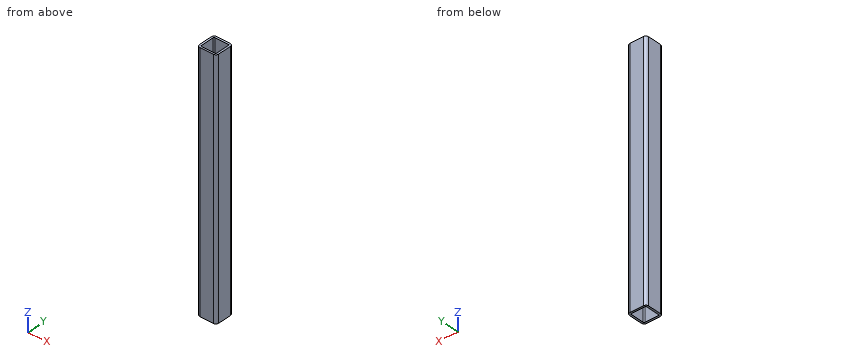
Autodesk Inventor part; units mm, degrees
ref_plane "Start Plane" through (0, 0, 10) normal (0, 0, 1) x (1, 0, 0)
ref_plane "End Plane" through (0, 0, 270) normal (0, 0, 1) x (1, 0, 0)
ref_plane "Work Plane4" through (167.5, -7, 270) normal (0, 0, 1) x (1, 0, 0)
ref_plane "Start Plane" through (0, 0, 10) normal (0, 0, 1) x (1, 0, 0)
ref_plane "End Plane" through (0, 0, 270) normal (0, 0, 1) x (1, 0, 0)
sketch "Sketch" plane through (0, 0, 0) normal (0, 0, 1) x (1, 0, 0)
  line L0 (-10, -7) -> (-10, 7)
  line L1 (-7, 10) -> (7, 10)
  line L2 (10, 7) -> (10, -7)
  line L3 (7, -10) -> (-7, -10)
  arc A0 (-10, -7) -> (-7, -10) centre (-7, -7) ccw
  arc A1 (-7, 10) -> (-10, 7) centre (-7, 7) ccw
  arc A2 (10, 7) -> (7, 10) centre (7, 7) ccw
  arc A3 (7, -10) -> (10, -7) centre (7, -7) ccw
  arc A4 (-7, 8) -> (-8, 7) centre (-7, 7) ccw
  line L4 (-7, 8) -> (7, 8)
  arc A5 (8, 7) -> (7, 8) centre (7, 7) ccw
  line L5 (8, 7) -> (8, -7)
  arc A6 (7, -8) -> (8, -7) centre (7, -7) ccw
  line L6 (7, -8) -> (-7, -8)
  arc A7 (-8, -7) -> (-7, -8) centre (-7, -7) ccw
  line L7 (-8, -7) -> (-8, 7)
  line L8 (0, 14.8698) -> (0, -14.8698) construction
  line L9 (-14.8698, 0) -> (14.8698, 0) construction
  dimension "d7" = 3
  dimension "d10" = 20
  dimension "d11" = 20
  dimension "d12" = 2
  dimension "d15" = 10
  dimension "d16" = 10
extrude "Body" add sketch "Sketch" along normal up to surface (260 mm away) from surface at 10
sketch "Sketch3" plane through (0, 0, 0) normal (0, 0, 1) x (1, 0, 0)
  line L0 (0, 0) -> (10, 0)
ref_plane "Work Plane3" through (0, 0, 0) normal (0, -1, 0) x (1, 0, 0)
sketch "Sketch4" plane through (0, 0, 0) normal (0, -1, 0) x (1, 0, 0)
  line L0 (-2, 10) -> (12, 10)
  line L1 (-2, 270) -> (12, 270)
  dimension "d18" = 260
ref_plane "Work Plane4" through (167.5, -7, 270) normal (0, 0, 1) x (1, 0, 0)
split "Split1" plane through (167.5, -7, 270) removes the side toward (0, 0, 1)
ref_plane "Work Plane5" through (-75, -7, 10) normal (0, 0, -1) x (-1, 0, 0)
split "Split2" plane through (-75, -7, 10) removes the side toward (0, 0, -1)
equation "\"d7\" = G_IR"
equation "\"d10\" = G_H"
equation "\"d11\" = G_W"
equation "\"d12\" = G_T"
equation "\"d15\" = 0.5 * d10"
equation "\"d16\" = 0.5 * d11"
equation "\"d3\" = G_L"
equation "\"G_W\" = 20"
equation "\"G_H\" = 20"
equation "\"G_T\" = 2"
equation "\"G_IR\" = 3"
equation "\"G_L\" = d18"
properties part number "ISO 12633-2 - 20x20x2 - 260" material "Steel, Mild"
The model under review builds one solid part; all positions refer to its coordinate system, in mm. Give positions to 0.01 mm unless a question says otherwise; leave off trailing zeros. Order: outer loops, then holes, each group sorted by start corner. A loop starts at its lowest first (then second) coordinate and runs counter-clockwise, first axis right, second up. Notation, with made-up numbers: (0, 24.25) - (11, 24.25) arc R12 cw to (11, 45.25) - close; hole circle Ø11 at (42.5, 42.5). An arc over 180 degrees is marked (long way). Use CSV: the item, a comma, the result in double quotes. Start each with the question number.
Q1. We need section A-A, the plane x = -3.75. Write out the cut boundary in (y, z), and give its area (3 significant figures).
Q2. We need section C-C, the plane z = 218. Write out the cut boundary in (x, y).
Q3. To check wall thickness, follow line 1 along Y through (x, z) = (4.5, 92.5); line 2 along X through (y, z) = (-7.5, 240.5). State the ranges of each line that lie inside material, in increasing order. Write a range as [from, to].
Outcome:
1,outline,"(-10, 10) - (-8, 10) - (-8, 270) - (-10, 270) - close; (8, 10) - (10, 10) - (10, 270) - (8, 270) - close"
1,area,"1,040 mm^2"
2,outline,"(-10, -7) arc R3 ccw to (-7, -10) - (7, -10) arc R3 ccw to (10, -7) - (10, 7) arc R3 ccw to (7, 10) - (-7, 10) arc R3 ccw to (-10, 7) - close; hole (-8, -7) arc R1 ccw to (-7, -8) - (7, -8) arc R1 ccw to (8, -7) - (8, 7) arc R1 ccw to (7, 8) - (-7, 8) arc R1 ccw to (-8, 7) - close"
3,line 1,"y = [-10, -8], [8, 10]"
3,line 2,"x = [-9.96, -7.87], [7.87, 9.96]"
